Build history of the part. All positions in model axes, mm. A direction names the side the tool comes from. Coordinates: 2 decimals unless noted, no trailing zeros. Loops run counter-clockwise (first coordinate to the right, second up) from the corner with the lowest first, then second, coordinate; pieces in that order, holes last. Notation, with made-up numbers: M 43.25,83.5 L 57.25,83.5 A17 cw 57.25,110.5 Z; hole C 15.25,8.25 d8. An arc over 180 degrees is marked long. Write each question's results on one line, items separated by ' | '. Start each with the question number.
from build123d import *

# Parameters (mm, degrees)
BOSS_EXTRUDE1_DEPTH = 175
CUT_EXTRUDE1_REACH  = 356.295
LPATTERN1_COUNT     = 4
LPATTERN1_PITCH     = 70
FILLET1_R           = 5


with BuildPart() as part:
    # Sketch1 → Boss-Extrude1 (new, symmetric)
    with BuildSketch(Plane.XY):
        Polygon((0, 300), (0, 0), (70, 0), (70, 10), (10, 10), (10, 290), (50, 290), (50, 300), align=None)
    extrude(amount=BOSS_EXTRUDE1_DEPTH, both=True)

    # Sketch2 → Cut-Extrude1 (cut, up to next)
    with BuildSketch(Plane(origin=(0, 300, 0), x_dir=(1, 0, 0), z_dir=(0, 1, 0)), mode=Mode.PRIVATE) as cut_extrude1_sk1:
        with BuildLine():
            Line((35, 115), (50, 115))
            Line((50, 115), (50, 95))
            Line((50, 95), (35, 95))
            ThreePointArc((35, 95), (25, 105), (35, 115))
        make_face()
    cut_extrude1_tool1 = extrude(cut_extrude1_sk1.sketch, amount=-CUT_EXTRUDE1_REACH, mode=Mode.PRIVATE) & part.part
    cut_extrude1 = cut_extrude1_tool1.solids().sort_by_distance((38.464021, 300, -105))[0]
    add(cut_extrude1, mode=Mode.SUBTRACT)

    # LPattern1: Cut-Extrude1 ×4
    with Locations(*[(0, 0, i * LPATTERN1_PITCH) for i in range(1, LPATTERN1_COUNT)]):
        add(cut_extrude1, mode=Mode.SUBTRACT)

    # Fillet1
    fillet1_edges = [part.edges().sort_by_distance(p)[0] for p in [
        (0, 0, 0),
        (0, 300, 0),
    ]]
    fillet(fillet1_edges, radius=FILLET1_R)


solid = part.part
1. Band-saw the part on A-A, the plane z = 73.5. List the corners of the cut face in (x, y).
2. Band-saw the part on B-B, the plane x = 30.5. List the corners of the cut face in (y, z), plus the area to 3 significant figures.
3. Band-saw the part on D-D, the plane z = -105. List the corners of the cut face in (x, y), plus the area to 3 significant figures.
4. Which spindle directions (+Z, -Z, +X, -X, +Y, -Y) get a long thin tool onto all of the face, cutting with end or side? Do faces 5 (the flat face through (40, 10, 2)), 6 (the flat face through (50, 295, 145)), 7 (the flat face through (42, 295, -115)). Say none if no direction does.
5. Wall check: line 1 along Y through (x, z) = (32, -94); line 2 along X through (y, z) = (186, -56). Give the ranges that are in metal, low to high.
6. Pin check, flat tips, straight feed: pin 1 (5 mm diameter, centred on y = 294.5, z = 65.5, fed in from +X); pin 2 (10 mm diameter, centred on y = 33.5, z = 83.5, fed in from +X); pin 3 (1.5 mm diameter, centred on x = 38.5, z = -32, fed in from +Y). Stop position of each tip, or through.
7. Band-saw the part on C-C, the plane y = 224.5. List the corners of the cut face in (x, z), plus the area to 3 significant figures.
8. Mould opens along Z. For faces 1 (the flat face through (43, 295, -95)), 2 (the flat face through (43, 295, 115)), 3 (the flat face through (28, 300, 2)), 4 (the flat face through (6, 140, 175)) say: +Z half, -Z half, draft (parallel to the pull), parting line (faces both ways), or undercut.
Checked values:
1) outline: M 0,5 A5 ccw 5,0 L 70,0 L 70,10 L 10,10 L 10,290 L 50,290 L 50,300 L 5,300 A5 ccw 0,295 Z
2) outline: M 0,-175 L 10,-175 L 10,175 L 0,175 Z; M 290,-175 L 300,-175 L 300,-113.93 L 290,-113.93 Z; M 290,-96.07 L 300,-96.07 L 300,-43.93 L 290,-43.93 Z; M 290,-26.07 L 300,-26.07 L 300,26.07 L 290,26.07 Z; M 290,43.93 L 300,43.93 L 300,96.07 L 290,96.07 Z; M 290,113.93 L 300,113.93 L 300,175 L 290,175 Z | area: 6,290 mm²
3) outline: M 0,5 A5 ccw 5,0 L 70,0 L 70,10 L 10,10 L 10,290 L 25,290 L 25,300 L 5,300 A5 ccw 0,295 Z | area: 3,740 mm²
4) face 5: +Z, -Z, +X | face 6: +Z, -Z, +X, +Y | face 7: +X, +Y
5) line 1: 0 to 10, 290 to 300 | line 2: 0 to 10
6) pin 1: x = 50 | pin 2: x = 10 | pin 3: y = 10
7) outline: M 0,-175 L 10,-175 L 10,175 L 0,175 Z | area: 3,500 mm²
8) face 1: undercut | face 2: undercut | face 3: draft | face 4: +Z half
